The listing builds one solid part. Answer for the finished solid, in the listing's coordinates (mm). Face numbers are marked on the shaded views. A direction names the side the tool comes from. Coordinates: 2 decimals unless noted, no trailing zeros. Order: outer loops, then holes, each group sorted by start corner. A loop starts at its lowest first (then second) coordinate and runs counter-clockwise, first axis right, second up. Notation, with made-up numbers: M 45.25,-11.75 L 59.25,-11.75 A10 ccw 59.25,-1.75 Z; hole C 68.25,80 d11. An arc over 180 degrees is marked long. One line per item, written item: value. Start each with the question number.
Q1. The part is cut by section D-D on y = -4. Give the vertices of the cut face in (x, z).
Q2. Each of these flat-tipped pins is pushed along its axis until it touches: pin 1 Ø0.8 at (x, z) = (-1, 3) entering from +Y; pin 2 Ø7 at (x, y) = (4.5, 0) entering from +Z; pin 3 Ø1 at (y, z) = (-5, 4) entering from +X. Where does it stop, or does it pass through?
Q3. The part is cut by section A-A on y = 2. Give the vertices of the cut face in (x, z), then the cut area to 3 significant figures.
Q4. The part is cut by section B-B on x = -9.75. Give the vertices of the cut face in (y, z), then the cut area to 3 significant figures.
Q5. Straight lines are drawn through the part: line 1 along Y through (x, z) = (2.5, 1.5); line 2 along Z through (x, y) = (5.5, 3); line 3 along X through (y, z) = (-0.25, 1.75). For each, find the intervals that lie inside material, in ascending order. Write a range as [from, to].
Q6. The part is cut by section C-C on z = 3. Give the vertices of the cut face in (x, y).
Q7. For the marked faces 1, 2 and 3, determine the directions among +Z, -Z, +X, -X, +Y, -Y from which every point of the face is accessible in a straight line to the end or side of a thin tool.
```python
from build123d import *

# Parameters (mm, degrees)
SKETCH1_W           = 24.8412
SKETCH1_H           = 23.6855
BOSS_EXTRUDE1_DEPTH = 1.0287
SKETCH2_W           = 8.5852
SKETCH2_H           = 8.5852
BOSS_EXTRUDE2_DEPTH = 2.8194
SKETCH3_R           = 3.429
BOSS_EXTRUDE3_DEPTH = 2.286


with BuildPart() as part:
    # Sketch1 → Boss-Extrude1 (new body)
    with BuildSketch(Plane.XY):
        Rectangle(SKETCH1_W, SKETCH1_H)
    extrude(amount=BOSS_EXTRUDE1_DEPTH)

    # Sketch2 → Boss-Extrude2 (add)
    with BuildSketch(Plane.XY.offset(1.0287)):
        with Locations((0.3683, -1.70815)):
            Rectangle(SKETCH2_W, SKETCH2_H)
    extrude(amount=BOSS_EXTRUDE2_DEPTH)

    # Sketch3 → Boss-Extrude3 (add)
    with BuildSketch(Plane.XY.offset(3.8481)):
        with Locations((0.3683, -1.70815)):
            Circle(SKETCH3_R)
    extrude(amount=BOSS_EXTRUDE3_DEPTH)


solid = part.part
```
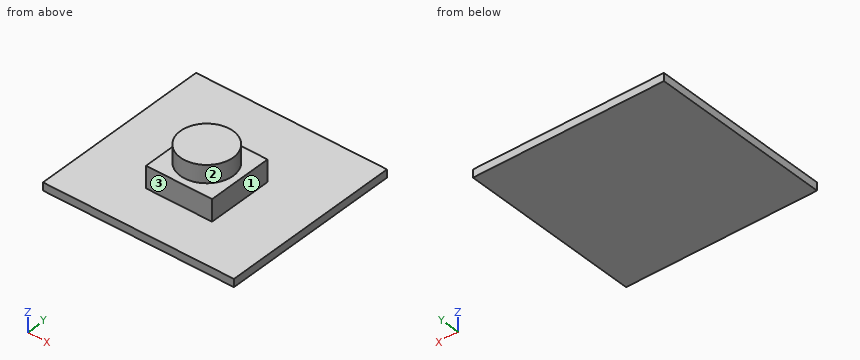
Output:
1. outline: M -12.42,0 L 12.42,0 L 12.42,1.03 L 4.66,1.03 L 4.66,3.85 L 2.92,3.85 L 2.92,6.13 L -2.18,6.13 L -2.18,3.85 L -3.92,3.85 L -3.92,1.03 L -12.42,1.03 Z
2. pin 1: stops at y = 2.58
2. pin 2: stops at z = 6.13
2. pin 3: stops at x = 4.66
3. outline: M -12.42,0 L 12.42,0 L 12.42,1.03 L 4.66,1.03 L 4.66,3.85 L -3.92,3.85 L -3.92,1.03 L -12.42,1.03 Z
3. area: 49.8 mm^2
4. outline: M -11.84,0 L 11.84,0 L 11.84,1.03 L -11.84,1.03 Z
4. area: 24.4 mm^2
5. line 1: y = [-6, 2.58]
5. line 2: z = [0, 1.03]
5. line 3: x = [-3.92, 4.66]
6. outline: M -3.92,-6 L 4.66,-6 L 4.66,2.58 L -3.92,2.58 Z
7. face 1: +Z, +X, +Y, -Y
7. face 2: +Z
7. face 3: +Z, +X, -X, -Y
